Work out the finished part from the listing and answer in its coordinate system (mm). A direction names the side the tool comes from. Round coordinates to 2 decimals unless told otherwise and drop trailing zeros. Loops run counter-clockwise (first coordinate to the right, second up) from the corner with the lowest first, then second, coordinate; pieces in that order, holes last.
```python
from build123d import *

# Parameters (mm, degrees)
SKETCH1_W              = 250
SKETCH1_H              = 120
BOSS_EXTRUDE1_DEPTH    = 100
CUT_EXTRUDE1_DEPTH     = 100
SKETCH5_W              = 20
SKETCH5_H              = 100
BOSS_EXTRUDE2_DEPTH    = 100
SKETCH6_W              = 20
SKETCH6_H              = 100
BOSS_EXTRUDE3_DEPTH    = 100
CUT_EXTRUDE2_START     = -100
CUT_EXTRUDE2_OUTLINE_R = 30
CUT_EXTRUDE2_DEPTH     = 100


# Read off the part's stored shape, not the designer's step: Cut-Extrude2
with BuildPart() as part:
    # Sketch1 → Boss-Extrude1 (new body)
    with BuildSketch(Plane(origin=(0, 0, 0), x_dir=(1, 0, 0), z_dir=(0, 1, 0))):
        with Locations((-125, 60)):
            Rectangle(SKETCH1_W, SKETCH1_H)
    extrude(amount=BOSS_EXTRUDE1_DEPTH)

    # Sketch2 → Cut-Extrude1 (cut)
    with BuildSketch(Plane(origin=(0, 100, 0), x_dir=(1, 0, 0), z_dir=(0, 1, 0))):
        with BuildLine():
            Line((-137.886107131, 60), (-250, 60))
            Line((-250, 60), (-250, 20))
            Line((-250, 20), (-217.607466681, 20))
            Line((-217.607466681, 20), (-177.886107131, 20))
            ThreePointArc((-177.886107131, 20), (-149.601835883, 31.715728753), (-137.886107131, 60))
        make_face()
        with BuildLine():
            Line((-250, 100), (-250, 60))
            Line((-250, 60), (-137.886107131, 60))
            ThreePointArc((-137.886107131, 60), (-149.601835883, 88.284271247), (-177.886107131, 100))
            Line((-177.886107131, 100), (-217.607466681, 100))
            Line((-217.607466681, 100), (-250, 100))
        make_face()
        with BuildLine():
            Line((0, 0), (0, 30))
            Line((0, 30), (-97.387762778, 30))
            ThreePointArc((-97.387762778, 30), (-115.851486425, 26.466018864), (-131.705192029, 16.363636364))
            ThreePointArc((-131.705192029, 16.363636364), (-150.729638754, 4.240777363), (-172.886107131, 0))
            Line((-172.886107131, 0), (0, 0))
        make_face()
        with BuildLine():
            Line((-97.387762778, 90), (0, 90))
            Line((0, 90), (0, 120))
            Line((0, 120), (-172.886107131, 120))
            ThreePointArc((-172.886107131, 120), (-150.729638754, 115.759222637), (-131.705192029, 103.636363636))
            ThreePointArc((-131.705192029, 103.636363636), (-115.851486425, 93.533981136), (-97.387762778, 90))
        make_face()
    extrude(amount=-CUT_EXTRUDE1_DEPTH, mode=Mode.SUBTRACT)

    # Sketch5 → Boss-Extrude2 (add)
    with BuildSketch(Plane.ZY.offset(250)):
        with Locations((-110, 50)):
            Rectangle(SKETCH5_W, SKETCH5_H)
    extrude(amount=BOSS_EXTRUDE2_DEPTH)

    # Sketch6 → Boss-Extrude3 (add)
    with BuildSketch(Plane.ZY.offset(250)):
        with Locations((-10, 50)):
            Rectangle(SKETCH6_W, SKETCH6_H)
    extrude(amount=BOSS_EXTRUDE3_DEPTH)

    # Cut-Extrude2 outline → Cut-Extrude2 (cut)
    with BuildSketch(Plane.XY.offset(CUT_EXTRUDE2_START)):
        with BuildLine():
            ThreePointArc((-266.908391633, 12.482609105), (-281.440890736, 3.537211244), (-298.135255344, 0))
            Line((-298.135255344, 0), (-172.886107131, 0))
            Line((-172.886107131, 0), (-172.886107131, 25))
            Line((-172.886107131, 25), (-233.816791268, 25))
            ThreePointArc((-233.816791268, 25), (-251.506753743, 21.766069191), (-266.908391633, 12.482609105))
        make_face()
        with BuildLine():
            Line((-350, 100), (-350, 50))
            ThreePointArc((-350, 50), (-320.568029043, 95.538875256), (-266.947820205, 87.482618173))
            ThreePointArc((-266.947820205, 87.482618173), (-251.561022849, 78.224637407), (-233.895648402, 75))
            Line((-233.895648402, 75), (-172.886107131, 75))
            Line((-172.886107131, 75), (-172.886107131, 100))
            Line((-172.886107131, 100), (-350, 100))
        make_face()
        with BuildLine():
            ThreePointArc((-301.864744656, 0), (-335.996534658, 15.262911764), (-350, 49.930454547))
            Line((-350, 49.930454547), (-350, 0))
            Line((-350, 0), (-301.864744656, 0))
        make_face()
        with Locations((-300, 49.965227274)):
            Circle(CUT_EXTRUDE2_OUTLINE_R)
    extrude(amount=CUT_EXTRUDE2_DEPTH, mode=Mode.SUBTRACT)


solid = part.part
```
1. Find section D-D (x = -163.5). Write down the section's boundary in (y, z).
Answer key:
outline: (0, -119.26) - (100, -119.26) - (100, -97.32) - (0, -97.32) - close; (0, -22.68) - (100, -22.68) - (100, -0.74) - (0, -0.74) - close
2. Which of the six approach directions +Z, -Z, +X, -X, +Y, -Y give full straight-line access (tool end or side, diameter ignored) to faces 1 (the face through (-263, 49, -20)), 2 (the face through (-203, 25, -10)), 3 (the face through (-323.8, 31.7, -10.1))?
Answer key:
face 1: -X, +Y, -Y
face 2: +Z, -Y
face 3: +Z
3. Given pin 1 (1 mm diameter, centred on x = -232.5, y = 59.5, fed in from +Z); pin 2 (22.5 mm diameter, centred on y = 8, z = -9.5, fed in from -X); pin 3 (16.5 mm diameter, centred on x = -215, z = -10, fed in from +Y); pin 4 (3 mm diameter, centred on x = -292.5, z = -15, fed in from -Y), each flat-ended and moving along its own axis, determine where each tip first touches the part or whether it passes through.
Answer key:
pin 1: stops at z = 0
pin 2: stops at x = -339.45
pin 3: stops at y = 75
pin 4: stops at y = 0.33
4. Find section A-A (x = -206). Write down the section's boundary in (y, z), then the cut area to 3 significant figures.
Answer key:
outline: (0, -120) - (100, -120) - (100, -100) - (0, -100) - close; (25, -20) - (75, -20) - (75, 0) - (25, 0) - close
area: 3,000 mm2
5. Determine the mould class of faces 4 (the face through (-134, 0, -74)), 5 (the face through (-251.27, 21.855, -10.14)), 6 (the face through (-115.61, 50.7, -26.56)) for opening direction X: +X half, -X half, draft (parallel to the pull), parting line (faces both ways), or undercut.
Answer key:
face 4: draft
face 5: undercut
face 6: +X half
6. Consider probe 1 along Z at (x, y) = (-270, 28.5); probe 2 along Y at (x, z) = (-300, -6.5); probe 3 along Z at (x, y) = (-313, 51). Determine where each line is inside the solid, lowest interval first.
Answer key:
probe 1: z = -120 to -100, -20 to 0
probe 2: y = 0 to 19.97, 79.97 to 99.97
probe 3: z = -120 to -100
7. Find section C-C (y = 93). Write down the section's boundary in (x, z), then the cut area to 3 significant figures.
Answer key:
outline: (-350, -120) - (-172.89, -120) arc R60 ccw to (-131.71, -103.64) arc R50 cw to (-97.39, -90) - (0, -90) - (0, -30) - (-97.39, -30) arc R50 cw to (-131.71, -16.36) arc R60 ccw to (-172.89, 0) - (-172.89, -20.31) arc R40 cw to (-172.89, -99.69) - (-172.89, -100) - (-350, -100) - close; (-325.46, -20) - (-274.54, -20) - (-274.54, 0) - (-325.46, 0) - close
area: 15,200 mm2
8. Find section B-B (y = 60). Write down the section's boundary in (x, z), then the cut area to 3 significant figures.
Answer key:
outline: (-350, -120) - (-172.89, -120) arc R60 ccw to (-131.71, -103.64) arc R50 cw to (-97.39, -90) - (0, -90) - (0, -30) - (-97.39, -30) arc R50 cw to (-131.71, -16.36) arc R60 ccw to (-172.89, 0) - (-271.73, 0) - (-271.73, -20) - (-177.89, -20) arc R40 cw to (-177.89, -100) - (-350, -100) - close; (-348.98, -20) - (-328.27, -20) - (-328.27, 0) - (-348.98, 0) - close
area: 16,500 mm2
